Job drawing, mm, ordinate dimensions from the low corner. One solid piece. Round coordinates to 2 decimals unless told otherwise and drop trailing zeros. Loops run counter-clockwise (first coordinate to the right, second up) from the corner with the lowest first, then second, coordinate; pieces in that order, holes last. Notation, with made-up numbers: (36.5, 83.25) - (41.5, 83.25) arc R18 cw to (41.5, 102.25) - close; hole circle Ø4 at (15.5, 59). An arc over 180 degrees is marked (long way). Answer as CSV lines item,"result". Start each with the question number.
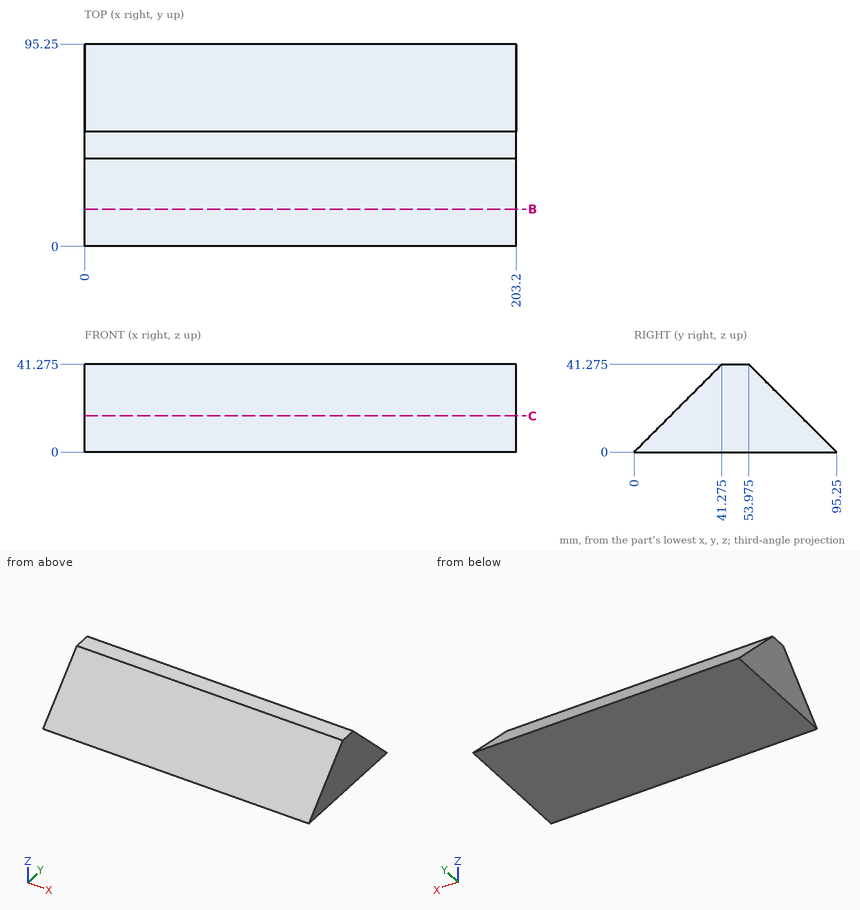
Q1. Pin check, flat tips, straight feed: pin 1 Ø8 at (x, z) = (88, 16) entering from -Y; pin 2 Ø1.5 at (x, z) = (160, 26.5) entering from +Y; pin 3 Ø1 at (x, z) = (125, 7.5) entering from +Y. Stop position of each tip, or through.
Q2. Band-saw the part on B-B, the plane y = 17.5. List the corners of the cut face in (x, z), then the cut area to 3 significant figures.
Q3. Wall check: probe 1 along Z at (x, y) = (92, 31.5); probe 2 along Y at (x, z) = (53.5, 37); probe 3 along Z at (x, y) = (55.5, 30.5). Give the ranges that are in metal, low to high. Write a range as [from, to].
Q4. Band-saw the part on C-C, the plane z = 17. List the corners of the cut face in (x, y), then the cut area to 3 significant figures.
Reported:
1,pin 1,"stops at y = 12"
1,pin 2,"stops at y = 69.5"
1,pin 3,"stops at y = 88.25"
2,outline,"(0, 0) - (203.2, 0) - (203.2, 17.5) - (0, 17.5) - close"
2,area,"3,560 mm2"
3,probe 1,"z = [0, 31.5]"
3,probe 2,"y = [37, 58.25]"
3,probe 3,"z = [0, 30.5]"
4,outline,"(0, 17) - (203.2, 17) - (203.2, 78.25) - (0, 78.25) - close"
4,area,"12,400 mm2"
